Answer from the drawing. Dimensions are ordinates in mm from the lowest x, y and z of the part. Round coordinates to 2 decimals unless told otherwise and drop trailing zeros. Order: outer loops, then holes, each group sorted by start corner. A loop starts at its lowest first (then second) coordinate and runs counter-clockwise, first axis right, second up. Notation, with made-up numbers: (34, -31) -> (85, -31) arc R29 ccw to (85, -7) -> close; hole circle Ø2 at (30, 13). An arc over 180 degrees is marked (long way). Use a Markdown table: item, result. Add a question column.
Item 1: A cutting plane is placed at C-C, the plane z = 50. Determine the outline of the cut face in (x, y) (1 decimal).
Item 2: A cutting plane is placed at B-B, the plane x = 31. Determine the outline of the cut face in (y, z).
Item 3: A cutting plane is placed at A-A, the plane y = 2.1. Determine the outline of the cut face in (x, z).
Item 4: Flat-ended cylindrical pins translate along their axes: P1, Ø1.5, axis at y = 2, z = 43.5, coming from the +X side; P2, Ø1.5, axis at x = 30.5, y = 2, coming from the -Z side; P3, Ø13.5, axis at x = 31, z = 9.5, coming from the -Y side; P4, Ø1, axis at x = 14, y = 0.5, coming from the -Z side (1 decimal). Find the tip coordinate at first contact, or state that the pin passes through.
Item 5: A cutting plane is placed at D-D, the plane x = 18. Determine the outline of the cut face in (y, z).
Item 6: Find the intervals of material crossed by L1, parallel to Z at x = 31, y = 2.1; L2, parallel to X at y = 0.6, z = 31; L3, parallel to X at y = 2.2, z = 20 (1 decimal), in increasing order. Write a range as [from, to].
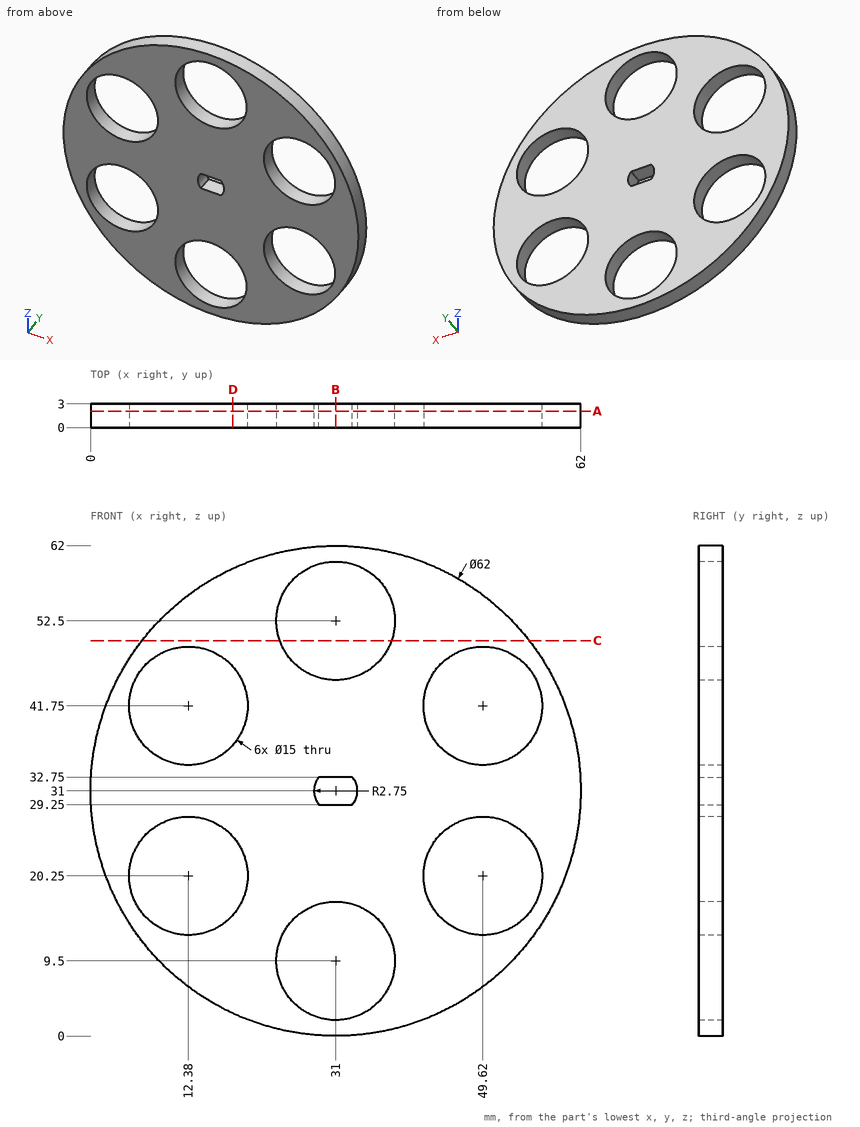
Reported:
| question | item | result |
|---|---|---|
| 1 | outline | (6.5, 0) -> (23.9, 0) -> (23.9, 3) -> (6.5, 3) -> close; (38.1, 0) -> (55.5, 0) -> (55.5, 3) -> (38.1, 3) -> close |
| 2 | outline | (0, 0) -> (3, 0) -> (3, 2) -> (0, 2) -> close; (0, 17) -> (3, 17) -> (3, 29.25) -> (0, 29.25) -> close; (0, 32.75) -> (3, 32.75) -> (3, 45) -> (0, 45) -> close; (0, 60) -> (3, 60) -> (3, 62) -> (0, 62) -> close |
| 3 | outline | circle Ø62 at (31, 31); hole circle Ø15 at (12.38, 20.25); hole circle Ø15 at (12.38, 41.75); hole circle Ø15 at (31, 9.5); hole circle Ø15 at (31, 52.5); hole (28.88, 29.25) -> (33.12, 29.25) arc R2.75 ccw to (33.12, 32.75) -> (28.88, 32.75) arc R2.75 ccw to start; hole circle Ø15 at (49.62, 20.25); hole circle Ø15 at (49.62, 41.75) |
| 4 | P1 | x = 59.69 |
| 4 | P2 | z = 0 |
| 4 | P3 | through |
| 4 | P4 | z = 4.8 |
| 5 | outline | (0, 2.86) -> (3, 2.86) -> (3, 15.28) -> (0, 15.28) -> close; (0, 25.22) -> (3, 25.22) -> (3, 36.78) -> (0, 36.78) -> close; (0, 46.72) -> (3, 46.72) -> (3, 59.14) -> (0, 59.14) -> close |
| 6 | L1 | [0, 2], [17, 29.25], [32.75, 45], [60, 62] |
| 6 | L2 | [0, 28.25], [33.75, 62] |
| 6 | L3 | [2, 4.9], [19.9, 42.1], [57.1, 60] |
